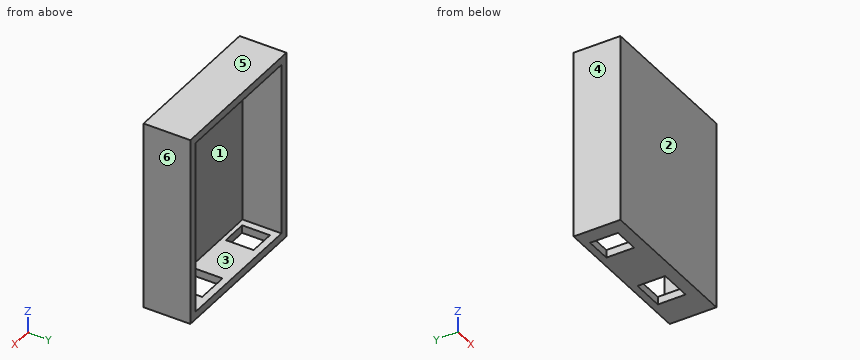
Autodesk Inventor part; units mm, degrees
ref_plane "YZ Plane" through (0, 0, 0) normal (1, 0, 0) x (0, 1, 0)
ref_plane "XZ Plane" through (0, 0, 0) normal (0, 1, 0) x (-1, 0, 0)
ref_plane "XY Plane" through (0, 0, 0) normal (0, 0, 1) x (1, 0, 0)
sketch "Sketch2" plane through (0, 0, 0) normal (0, 1, 0) x (-1, 0, 0)
  line L0 (0, 0) -> (-59, 0)
  line L1 (-59, 0) -> (-59, 73)
  line L2 (-59, 73) -> (0, 73)
  line L3 (0, 73) -> (0, 0)
  dimension "d0" = 59
  dimension "d1" = 73
extrude "Extrusion1" add sketch "Sketch2" along normal blind 18
shell "Shell1" thickness 3 removed faces 1 at (19.6667, 18, 24.3333)
sketch "Sketch3" plane through (59, 0, 0) normal (0, 0, -1) x (-1, 0, 0)
  line L0 (11.5, 15.35) -> (24, 15.35)
  line L1 (24, 15.35) -> (24, 4.65)
  line L2 (24, 4.65) -> (11.5, 4.65)
  line L3 (11.5, 4.65) -> (11.5, 15.35)
  line L4 (0, 0) -> (0, 18)
  line L5 (0, 0) -> (59, 0)
  line L6 (43.1, 15.35) -> (53.1, 15.35)
  line L7 (53.1, 15.35) -> (53.1, 4.65)
  line L8 (53.1, 4.65) -> (43.1, 4.65)
  line L9 (43.1, 4.65) -> (43.1, 15.35)
  line L10 (59, 0) -> (59, 18)
  dimension "d5" = 11.5
  dimension "d6" = 4.65
  dimension "d7" = 12.5
  dimension "d8" = 10.7
  dimension "d10" = 10
  dimension "d11" = 10.7
  dimension "d12" = 4.65
  dimension "d16" = 43.1
extrude "Extrusion2" cut sketch "Sketch3" against normal blind 30
equation "\"d11\" = d8"
equation "\"d12\" = d6"
properties part number "arduino array box v02"
Verification items for the finished model (mm, model axes). Face numbers are marked on the shaded views. A direction names the side the tool comes from. Coordinates: 2 decimals unless noted, no trailing zeros. Order: outer loops, then holes, each group sorted by start corner. A loop starts at its lowest first (then second) coordinate and runs counter-clockwise, first axis right, second up. Notation, with made-up numbers: (0.25, 70) -> (49.25, 70) arc R17 ccw to (49.25, 101) -> close; hole circle Ø7 at (21, 64). An arc over 180 degrees is marked (long way). Put each result on its own line as item: value. Start each with the question number.
1. Cross-section at D-D, the plane x = 49. Record the boundary of the cut face in (y, z).
2. Cross-section at B-B, the plane x = 43. Record the boundary of the cut face in (y, z), then the cut area to 3 significant figures.
3. Access from +Z, -Z, +X, -X, +Y, -Y to the whole of each face (thin tool, end or side, straight path). Record for the marked faces 1 and 2.
4. Cross-section at A-A, the plane y = 9. Record the boundary of the cut face in (x, z).
5. Go/stop test with flat-tipped pins: pin 1 Ø2 at (x, y) = (7.5, 8) entering from -Z; pin 2 Ø16 at (x, z) = (37, 52) entering from +Y. Record where each tip stops, or that it passes through.
6. Mould release check, pull along X, two halves, no side actions. Record for the marked faces 3, 4, 5 and 6: released by +X, released by -X, zero draft, split by the parting line, or undercut.
7. Material ranges on L1, parallel to Z at x = 6, y = 3.75; L2, parallel to X at y = 15, z = 40; L3, parallel to Z at x = 9.5, y = 11.75, recorded low to high. Write a range as [from, to].
8. Cross-section at C-C, the plane z = 65.5. Record the boundary of the cut face in (x, y).
Computed:
1. outline: (0, 0) -> (18, 0) -> (18, 3) -> (3, 3) -> (3, 70) -> (18, 70) -> (18, 73) -> (0, 73) -> close
2. outline: (0, 0) -> (4.65, 0) -> (4.65, 3) -> (3, 3) -> (3, 70) -> (18, 70) -> (18, 73) -> (0, 73) -> close; (15.35, 0) -> (18, 0) -> (18, 3) -> (15.35, 3) -> close
2. area: 277 mm2
3. face 1: +Y
3. face 2: +Z, -Z, +X, -X, -Y
4. outline: (0, 0) -> (5.9, 0) -> (5.9, 3) -> (3, 3) -> (3, 70) -> (56, 70) -> (56, 3) -> (47.5, 3) -> (47.5, 0) -> (59, 0) -> (59, 73) -> (0, 73) -> close; (15.9, 0) -> (35, 0) -> (35, 3) -> (15.9, 3) -> close
5. pin 1: z = 70
5. pin 2: y = 3
6. face 3: undercut
6. face 4: released by -X
6. face 5: zero draft
6. face 6: released by +X
7. L1: [0, 3], [70, 73]
7. L2: [0, 3], [56, 59]
7. L3: [70, 73]
8. outline: (0, 0) -> (59, 0) -> (59, 18) -> (56, 18) -> (56, 3) -> (3, 3) -> (3, 18) -> (0, 18) -> close
